Autodesk Inventor part; units mm, degrees
ref_plane "Start Plane" through (0, 0, 19.05) normal (0, 0, 1) x (1, 0, 0)
ref_plane "End Plane" through (0, 0, 1149.35) normal (0, 0, 1) x (1, 0, 0)
ref_plane "Work Plane4" through (-6.35, -19.05, 19.05) normal (0, 0, -1) x (-1, 0, 0)
sketch "Caster Mount Pattern" plane through (0, 0, 0) normal (0, 0, 1) x (1, 0, 0)
  line L0 (-94.6641, 144.1787) -> (-56.5641, 144.1787) construction
  line L1 (-56.5641, 144.1787) -> (-56.5641, 67.9787) construction
  line L2 (-56.5641, 67.9787) -> (-94.6641, 67.9787) construction
  line L3 (-94.6641, 67.9787) -> (-94.6641, 144.1787) construction
  circle A0 centre (-94.6641, 144.1787) radius 3.175
  circle A1 centre (-56.5641, 144.1787) radius 3.175
  circle A2 centre (-56.5641, 67.9787) radius 3.175
  circle A3 centre (-94.6641, 67.9787) radius 3.175
  point P0 (-75.6141, 93.3787)
  dimension "d11" = 6.35
  dimension "d12" = 38.1
  dimension "d13" = 76.2
ref_plane "Start Plane" through (0, 0, 19.05) normal (0, 0, 1) x (1, 0, 0)
ref_plane "End Plane" through (0, 0, 1149.35) normal (0, 0, 1) x (1, 0, 0)
sketch "Sketch" plane through (0, 0, 0) normal (0, 0, 1) x (1, 0, 0)
  line L0 (-25.4, 12.7) -> (25.4, 12.7)
  line L1 (25.4, 12.7) -> (25.4, -12.7)
  line L2 (25.4, -12.7) -> (-25.4, -12.7)
  line L3 (-25.4, -12.7) -> (-25.4, 12.7)
  line L4 (22.225, 9.525) -> (-22.225, 9.525)
  line L5 (-22.225, 9.525) -> (-22.225, -9.525)
  line L6 (-22.225, -9.525) -> (22.225, -9.525)
  line L7 (22.225, -9.525) -> (22.225, 9.525)
  point P0 (0, 0)
  point P1 (0, 12.7)
  point P2 (-25.4, 0)
  dimension "d0" = 50.8
  dimension "d1" = 25.4
  dimension "d2" = 3.175
extrude "Body" add sketch "Sketch" along normal up to surface (1130.3 mm away) from surface at 19.05
sketch "Sketch2" plane through (0, 0, 0) normal (0, 0, 1) x (1, 0, 0)
  line L0 (0, 0) -> (10, 0)
ref_plane "Work Plane3" through (0, 0, 0) normal (0, -1, 0) x (1, 0, 0)
sketch "Sketch3" plane through (0, 0, 0) normal (0, -1, 0) x (1, 0, 0)
  line L0 (-2, 19.05) -> (12, 19.05)
  line L1 (-2, 1149.35) -> (12, 1149.35)
  dimension "d10" = 1130.3
ref_plane "Work Plane4" through (-6.35, -19.05, 19.05) normal (0, 0, -1) x (-1, 0, 0)
split "Split1" plane through (-6.35, -19.05, 19.05) removes the side toward (0, 0, -1)
ref_plane "Work Plane5" through (755.65, -19.05, 1149.35) normal (0, 0, 1) x (1, 0, 0)
split "Split2" plane through (755.65, -19.05, 1149.35) removes the side toward (0, 0, 1)
sketch "Sketch4" plane through (-25.4, -12.7, 19.05) normal (0, -1, 0) x (1, 0, 0)
  line L0 (50.8, 0) -> (0, 0)
  line L1 (50.8, 0) -> (50.8, 1130.3)
  line L2 (50.8, 1130.3) -> (0, 1130.3)
  line L3 (6.35, 101.6) -> (44.45, 101.6) construction
  line L4 (44.45, 101.6) -> (44.45, 25.4) construction
  line L5 (44.45, 25.4) -> (6.35, 25.4) construction
  line L6 (6.35, 25.4) -> (6.35, 101.6) construction
  circle A0 centre (6.35, 101.6) radius 3.175
  circle A1 centre (44.45, 101.6) radius 3.175
  circle A2 centre (44.45, 25.4) radius 3.175
  circle A3 centre (6.35, 25.4) radius 3.175
  line L7 (6.35, 603.25) -> (44.45, 603.25) construction
  line L8 (44.45, 603.25) -> (44.45, 527.05) construction
  line L9 (44.45, 527.05) -> (6.35, 527.05) construction
  line L10 (6.35, 527.05) -> (6.35, 603.25) construction
  circle A4 centre (6.35, 603.25) radius 3.175
  circle A5 centre (44.45, 603.25) radius 3.175
  circle A6 centre (44.45, 527.05) radius 3.175
  circle A7 centre (6.35, 527.05) radius 3.175
  line L11 (6.35, 1104.9) -> (44.45, 1104.9) construction
  line L12 (44.45, 1104.9) -> (44.45, 1028.7) construction
  line L13 (44.45, 1028.7) -> (6.35, 1028.7) construction
  line L14 (6.35, 1028.7) -> (6.35, 1104.9) construction
  circle A8 centre (6.35, 1104.9) radius 3.175
  circle A9 centre (44.45, 1104.9) radius 3.175
  circle A10 centre (44.45, 1028.7) radius 3.175
  circle A11 centre (6.35, 1028.7) radius 3.175
  point P0 (25.4, -19.05)
  point P1 (25.4, 101.6)
  point P2 (25.4, 527.05)
  point P3 (25.4, 603.25)
  point P4 (25.4, 1028.7)
  point P5 (25.4, 25.4)
  point P6 (25.4, 0)
  point P7 (50.8, 565.15)
  point P8 (44.45, 565.15)
  dimension "d14" = 25.4
  dimension "d15" = 25.4
extrude "Extrusion3" cut sketch "Sketch4" against normal up to surface (25.4 mm away)
equation "\"d15\" = d14"
equation "\"G_OFFSET_START\" = -19.05"
equation "\"G_OFFSET_END\" = -19.05"
equation "\"d5\" = -G_OFFSET_START"
equation "\"d6\" = length + G_OFFSET_END"
equation "\"G_L\" = 1130.3"
properties part number "2x1x.125 Tube" material "Aluminum-6061"
Verification items for the finished model (mm, model axes). A direction names the side the tool comes from. Round coordinates to 2 decimals unless told otherwise and drop trailing zeros. Write each loop counter-clockwise with the first axis right and the second up, starting at its lowest first coordinate (ties: lowest second). Pieces come first, ordered by that corner, then holes. Notation, with made-up numbers: (-37.5, 22.5) - (-9.5, 22.5) arc R17 cw to (-9.5, 48.5) - close; hole circle Ø2 at (38.5, -12.75). An arc over 180 degrees is marked (long way). Answer as a JSON object with one key per item and string values. Group by question number.
Q1. Thickness scan on line 1 (X direction, y = 10.7, z = 1123.95) (3 decimals); line 2 (Y direction, x = 13.5, z = 636) (3 decimals); line 3 (X direction, y = -2.5, z = 1064) (3 decimals). Record the ranges inside material, lowest first.
Q2. Section check B-B, the plane y = -3. Enter the section's corners in (x, z) (3 decimals).
Q3. Section check C-C, the plane z = 179. Enter the section's corners in (x, y) (3 decimals).
Q4. Tool access check on faces 1 (the flat face through (0, 12.7, 576)), 2 (the flat face through (0, 9.525, 576)). Record the directions out of +Z, -Z, +X, -X, +Y, -Y that give a thin tool (end or side, any length) a straight path to the whole face; none if there is none.
Q5. Section check A-A, the plane x = -3. Enter the section's corners in (y, z) (3 decimals).
Found:
{
 "1": {"line 1": "x = -25.4 to -22.225, -15.875 to 15.875, 22.225 to 25.4", "line 2": "y = -12.7 to -9.525, 9.525 to 12.7", "line 3": "x = -25.4 to -22.225, 22.225 to 25.4"},
 "2": {"outline": "(-25.4, 19.05) - (-22.225, 19.05) - (-22.225, 1149.35) - (-25.4, 1149.35) - close; (22.225, 19.05) - (25.4, 19.05) - (25.4, 1149.35) - (22.225, 1149.35) - close"},
 "3": {"outline": "(-25.4, -12.7) - (25.4, -12.7) - (25.4, 12.7) - (-25.4, 12.7) - close; hole (-22.225, -9.525) - (22.225, -9.525) - (22.225, 9.525) - (-22.225, 9.525) - close"},
 "4": {"face 1": "+Z, -Z, +X, -X, +Y", "face 2": "+Z, -Z"},
 "5": {"outline": "(-12.7, 19.05) - (-9.525, 19.05) - (-9.525, 1149.35) - (-12.7, 1149.35) - close; (9.525, 19.05) - (12.7, 19.05) - (12.7, 1149.35) - (9.525, 1149.35) - close"}
}
